Read the model definition and answer for the solid it produces. Units are mm, in the model's axes. A direction names the side the tool comes from. Round coordinates to 2 decimals unless told otherwise and drop trailing zeros. Order: outer loops, then holes, each group sorted by start corner. A loop starts at its lowest first (then second) coordinate and runs counter-clockwise, first axis right, second up. Notation, with made-up numbers: (65.5, 72.5) -> (91.5, 72.5) arc R19 ccw to (91.5, 82.5) -> close; hole circle Ø4 at (-21, -17.5). An arc over 180 degrees is marked (long way). Answer as a JSON object with one key per item and string values. Group by question number.
Item 1: Section D-D, the plane y = -16 is taken. Write down the section's boundary in (x, z), plus the area to 3 significant figures.
Item 2: The mould has two halves that part along Y. Classify faces 5 (the cylindrical face through (39.028, -1.051, 12.106)), 6 (the flat face through (37.5, 15, 13)), 7 (the cylindrical face through (27.6, 17.7, 16.1)), 8 (the flat face through (-28, 22, 13.1)): pulls with the +Y half, pulls with the -Y half, needs draft (parallel to the pull), parting line crosses it, or undercut.
Item 3: Given P1, Ø4, axis at y = 3.5, z = 5.5, coming from the -X side; P2, Ø9, axis at y = 15, z = 11.5, coming from the +X side; P3, Ø7, axis at x = 30, y = 19.5, coming from the -Z side; P4, Ø6.5, axis at x = 43.12, y = -15, coming from the +Z side, each flat-ended and moving along its own axis, determine where each tip first touches the part or whether it passes through.
Item 4: Section C-C, the plane y = 19.5 is taken. Count the separate pieces of the cut face and the enclosed holes in it, plus the area to 3 significant figures.
Item 5: Consider probe 1 along X at (y, z) = (19.5, 17.75); probe 2 along X at (y, z) = (19.5, 10.7); probe 3 along Y at (x, z) = (0, 16). Determine where each line is inside the solid, lowest interval first. Write a range as from..to.
Item 6: For faces 1 (the flat face through (0.2, -2.5, 1.7)), 2 (the flat face through (1, 12, 7.1)), 3 (the flat face through (-55, -15, 9)), 4 (the flat face through (32, 22, 13.1)), determine the directions among +Z, -Z, +X, -X, +Y, -Y from which every point of the face is accessible in a straight line to the end or side of a thin tool.
Item 7: Section B-B, the plane z = 14.75 is taken. Write down the section's boundary in (x, y), plus the area to 3 significant figures.
Item 8: Section A-A, the plane x = -30 is taken. Write down the section's boundary in (y, z), plus the area to 3 significant figures.
from build123d import *

# Parameters (mm, degrees)
F1_DEPTH = 19.1
F2_R     = 3
F3_DEPTH = 19.101
F4_R     = 5.5
F4_R_2   = 3
F5_DEPTH = 13.1
F7_DEPTH = 92.501
F8_R     = 4
F9_DEPTH = 19.101
F10_R    = 5.08
F11_R    = 5.08
F12_SIZE = 0.762


with BuildPart() as f1:
    # F0 (on Top) → F1 (new body)
    with BuildSketch(Plane.XY):
        Polygon((-55, -2.5), (-55, -27.5), (55, -27.5), (55, -2.5), (37.5, -2.5), (37.5, 27.5), (-37.5, 27.5), (-37.5, -2.5), align=None)
    extrude(amount=F1_DEPTH)

    # F2 (on face) → F3 (cut, through all)
    with BuildSketch(Plane.XY.offset(19.1)):
        with Locations((-30, 19.5)):
            Circle(F2_R)
        with Locations((0, 19.5)):
            Circle(F2_R)
        with Locations((30, 19.5)):
            Circle(F2_R)
    extrude(amount=-F3_DEPTH, mode=Mode.SUBTRACT)

    # F4 (on face) → F5 (cut)
    with BuildSketch(Plane(origin=(0, 0, 0), x_dir=(1, 0, 0), z_dir=(0, 0, -1))):
        with Locations((-30, -19.5)):
            Circle(F4_R)
        with Locations((-30, -19.5)):
            Circle(F4_R_2, mode=Mode.SUBTRACT)
        with Locations((0, -19.5)):
            Circle(F4_R)
        with Locations((0, -19.5)):
            Circle(F4_R_2, mode=Mode.SUBTRACT)
        with Locations((30, -19.5)):
            Circle(F4_R)
        with Locations((30, -19.5)):
            Circle(F4_R_2, mode=Mode.SUBTRACT)
    extrude(amount=-F5_DEPTH, mode=Mode.SUBTRACT)

    # F6 (on face) → F7 (cut, through all)
    with BuildSketch(Plane.YZ.offset(37.5)):
        Polygon((27.5, 7.1), (14.2632350326, 7.1), (-2.5, 7.1), (-2.5, 0), (27.5, 0), align=None)
    extrude(amount=-F7_DEPTH, mode=Mode.SUBTRACT)

    # F8 (on face) → F9 (cut, through all)
    with BuildSketch(Plane.XY.offset(19.1)):
        with Locations((-39.879388541, -15)):
            Circle(F8_R)
        with Locations((43.120611459, -15)):
            Circle(F8_R)
    extrude(amount=-F9_DEPTH, mode=Mode.SUBTRACT)

    # F10
    f10_edges = [f1.edges().sort_by_distance(p)[0] for p in [
        (55, -2.5, 9.55),
        (37.5, -2.5, 13.1),
        (-37.5, -2.5, 13.1),
        (-55, -2.5, 9.55),
        (55, -27.5, 9.55),
        (-55, -27.5, 9.55),
    ]]
    fillet(f10_edges, radius=F10_R)

    # F11
    f11_edges = [f1.edges().sort_by_distance(p)[0] for p in [
        (0, -2.5, 7.1),
    ]]
    fillet(f11_edges, radius=F11_R)

    # F12
    f12_edges = [f1.edges().sort_by_distance(p)[0] for p in [
        (0, -27.5, 19.1),
    ]]
    chamfer(f12_edges, length=F12_SIZE)


solid = f1.part
Values found:
{
 "1": {"outline": "(-55, 0) -> (-43.75, 0) -> (-43.75, 19.1) -> (-54.24, 19.1) -> (-55, 18.34) -> close; (-36.01, 0) -> (39.25, 0) -> (39.25, 19.1) -> (-36.01, 19.1) -> close; (46.99, 0) -> (55, 0) -> (55, 18.34) -> (54.24, 19.1) -> (46.99, 19.1) -> close", "area": "1,800 mm2"},
 "2": {"face 5": "pulls with the +Y half", "face 6": "needs draft", "face 7": "undercut", "face 8": "undercut"},
 "3": {"P1": "x = -37.51", "P2": "x = 37.5", "P3": "z = 13.1", "P4": "through"},
 "4": {"separate pieces": "4", "enclosed holes": "0", "area": "593 mm2"},
 "5": {"probe 1": "-37.5..-33, -27..-3, 3..27, 33..37.5", "probe 2": "-37.5..-35.5, -24.5..-5.5, 5.5..24.5, 35.5..37.5", "probe 3": "-27.5..16.5, 22.5..27.5"},
 "6": {"face 1": "-Z, +Y", "face 2": "-Z, +X, -X, +Y", "face 3": "+Z, -Z, -X, +Y, -Y", "face 4": "-Z"},
 "7": {"outline": "(-55, -22.42) arc R5.08 ccw to (-49.92, -27.5) -> (49.92, -27.5) arc R5.08 ccw to (55, -22.42) -> (55, -7.58) arc R5.08 ccw to (49.92, -2.5) -> (42.58, -2.5) arc R5.08 cw to (37.5, 2.58) -> (37.5, 27.5) -> (-37.5, 27.5) -> (-37.5, 2.58) arc R5.08 cw to (-42.58, -2.5) -> (-49.92, -2.5) arc R5.08 ccw to (-55, -7.58) -> close; hole circle Ø8 at (-39.88, -15); hole circle Ø6 at (-30, 19.5); hole circle Ø6 at (0, 19.5); hole circle Ø6 at (30, 19.5); hole circle Ø8 at (43.12, -15)", "area": "4,800 mm2"},
 "8": {"outline": "(-27.5, 0) -> (-2.5, 0) -> (-2.5, 2.02) arc R5.08 cw to (2.58, 7.1) -> (14, 7.1) -> (14, 13.1) -> (16.5, 13.1) -> (16.5, 19.1) -> (-26.74, 19.1) -> (-27.5, 18.34) -> close; (22.5, 13.1) -> (25, 13.1) -> (25, 7.1) -> (27.5, 7.1) -> (27.5, 19.1) -> (22.5, 19.1) -> close", "area": "741 mm2"}
}
